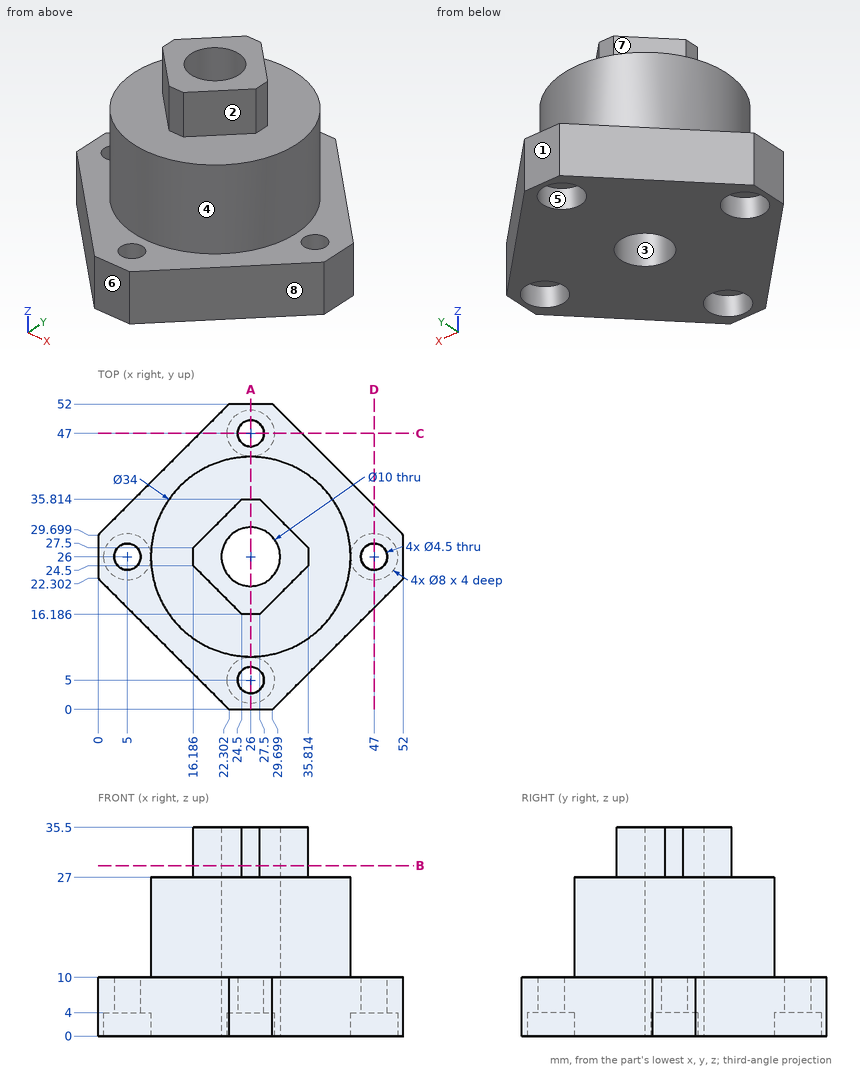
Can you work these out from the drawing? Everything is in mm from the part's minimum corner. A direction names the side the tool comes from. Round coordinates to 2 decimals unless told otherwise and drop trailing zeros. Loops run counter-clockwise (first coordinate to the right, second up) from the corner with the lowest first, then second, coordinate; pieces in that order, holes last. Notation, with made-up numbers: (-39.75, 20.5) -> (-29.75, 20.5) arc R24 cw to (-29.75, 58.5) -> close; hole circle Ø10 at (64.25, 56.25). An arc over 180 degrees is marked (long way). Answer in a Markdown table with one row per item.
Item 1: Will these pins go through, and if not, where does the flat tip stop? P1, Ø12, axis at x = 46.5, y = 20.5, coming from the +Z side; P2, Ø2, axis at y = 9, z = 10, coming from the +X side; P3, Ø2.5, axis at x = 5, y = 26, coming from the -Z side; P4, Ø0.9, axis at x = 26.5, z = 33, coming from the +Y side.
Answer block:
| item | result |
|---|---|
| P1 | z = 27 |
| P2 | x = 39.7 |
| P3 | through |
| P4 | y = 35.81 |
Item 2: Suppose I cut it at B-B, the plane z = 29. List the corners of the cut face in (x, y) for me.
Answer block:
| item | result |
|---|---|
| outline | (16.19, 24.5) -> (24.5, 16.19) -> (27.5, 16.19) -> (35.81, 24.5) -> (35.81, 27.5) -> (27.5, 35.81) -> (24.5, 35.81) -> (16.19, 27.5) -> close; hole circle Ø10 at (26, 26) |
Item 3: Suppose I cut it at C-C, the plane y = 47. List the corners of the cut face in (x, z) for me, plus the area to 3 significant figures.
Answer block:
| item | result |
|---|---|
| outline | (17.3, 0) -> (22, 0) -> (22, 4) -> (23.75, 4) -> (23.75, 10) -> (17.3, 10) -> close; (28.25, 4) -> (30, 4) -> (30, 0) -> (34.7, 0) -> (34.7, 10) -> (28.25, 10) -> close |
| area | 115 mm² |
Item 4: Suppose I cut it at A-A, the plane x = 26. Give the number of separate pieces and of enclosed holes in the cut face, plus the area to 3 significant figures.
Answer block:
| item | result |
|---|---|
| separate pieces | 4 |
| enclosed holes | 0 |
| area | 792 mm² |
Item 5: On a 3-axis mill with a long thin cutter (end or side, diameter ignored), from which of +Z, -Z, +X, -X, +Y, -Y can I reach the whole of each face in a straight line? I mean the marked faces 4, 5, 6, 7 and 8. Say none if no direction works.
Answer block:
| item | result |
|---|---|
| face 4 | +Z |
| face 5 | -Z |
| face 6 | +Z, -Z, +X, -X, -Y |
| face 7 | +Z, -X, +Y |
| face 8 | +Z, -Z, +X, -Y |
Item 6: We'd pull the mould along X, two halves only. Please class the marked faces 1, 2 and 3: released by +X, released by -X, zero draft, split by the parting line, or undercut.
Answer block:
| item | result |
|---|---|
| face 1 | zero draft |
| face 2 | released by +X |
| face 3 | undercut |
Item 7: If I drill on probe 1 along Y at (x, z) = (26, 2); probe 2 along X at (y, z) = (27.5, 9) (1 decimal); probe 3 along Z at (x, y) = (20, 16.5), over which ranges is the centre line in solid material (lowest first)?
Answer block:
| item | result |
|---|---|
| probe 1 | 0 to 1, 9 to 21, 31 to 43, 51 to 52 |
| probe 2 | 0 to 3.3, 6.7 to 21.2, 30.8 to 45.3, 48.7 to 52 |
| probe 3 | 0 to 27 |
